from build123d import *

# Parameters (mm, degrees)
F1_DEPTH = 2.54
F2_DEPTH = 5.08
F3_DEPTH = 7.62


with BuildPart() as f1:
    # F0 (on Top) → F1 (new body)
    with BuildSketch(Plane.XY):
        Polygon((-24.428534, 7.051245), (-30.778534, -3.947278), (-28.57883, -5.217278), (-24.428534, 1.971245), (-20.278239, -5.217278), (-18.078534, -3.947278), align=None)
    extrude(amount=F1_DEPTH)

    # F0 (on Top) → F2 (join)
    with BuildSketch(Plane.XY):
        Polygon((-24.428534, -12.4058), (-24.428534, -14.9458), (-11.728534, -14.9458), (-18.078534, -3.947278), (-20.278239, -5.217278), (-16.127943, -12.4058), align=None)
    extrude(amount=F2_DEPTH)

    # F0 (on Top) → F3 (join)
    with BuildSketch(Plane.XY):
        Polygon((-30.778534, -3.947278), (-37.128534, -14.9458), (-24.428534, -14.9458), (-24.428534, -12.4058), (-32.729125, -12.4058), (-28.57883, -5.217278), align=None)
    extrude(amount=F3_DEPTH)


solid = f1.part
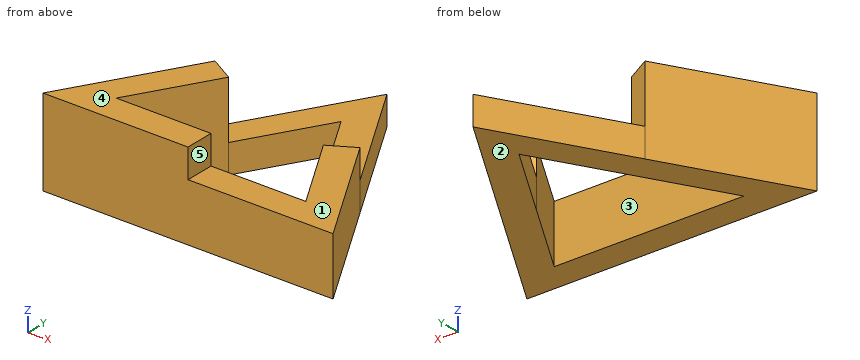
Model file for the job. Use its own axes, mm. Face numbers are marked on the shaded views. A direction names the side the tool comes from. Round coordinates to 2 decimals unless told otherwise and drop trailing zeros. Loops run counter-clockwise (first coordinate to the right, second up) from the corner with the lowest first, then second, coordinate; pieces in that order, holes last.
1. Band-saw the part on D-D, the plane z = 5.5. List the corners of the cut face in (x, y).
Check values:
outline: (-37.13, -14.95) - (-24.43, -14.95) - (-24.43, -12.41) - (-32.73, -12.41) - (-28.58, -5.22) - (-30.78, -3.95) - close
2. Tool access for the marked faces 1 and 2: list every direction of +Z, -Z, +X, -X, +Y, -Y with a clear straight run to the whole face (end or side of a thin tool).
Check values:
face 1: +Z, +X, +Y, -Y
face 2: -Z, +X, -X, +Y, -Y
3. Drop flat-ended pins along their axis: P1, Ø8, axis at x = -21, y = -7, coming from the +Z side; P2, Ø0.8, axis at y = -13.5, z = 6.5, coming from the +X side; P3, Ø4, axis at x = -26.5, z = 2.5, coming from the +Y side. Give the stop position or say it passes through.
Check values:
P1: stops at z = 5.08
P2: stops at x = -24.43
P3: stops at y = 6.93
4. Band-saw the part on C-C, the plane y = -2.5. List the corners of the cut face in (x, z), and give its area (3 significant figures).
Check values:
outline: (-29.94, 0) - (-27.01, 0) - (-27.01, 2.54) - (-29.94, 2.54) - close; (-21.85, 0) - (-18.91, 0) - (-18.91, 2.54) - (-21.85, 2.54) - close
area: 14.9 mm2
5. Wall check: probe 1 along Y at (x, z) = (-30, 1); probe 2 along Y at (x, z) = (-22, 3); probe 3 along Z at (x, y) = (-19.5, -2.75). Give the ranges that are in metal, low to high.
Check values:
probe 1: y = -14.95 to -12.41, -7.68 to -2.6
probe 2: y = -14.95 to -12.41
probe 3: z = 0 to 2.54
6. Band-saw the part on A-A, the plane x = -31.5. List the corners of the cut face in (y, z), and give its area (3 significant figures).
Check values:
outline: (-14.95, 0) - (-12.41, 0) - (-12.41, 7.62) - (-14.95, 7.62) - close; (-10.28, 0) - (-5.2, 0) - (-5.2, 7.62) - (-10.28, 7.62) - close
area: 58.1 mm2
7. Band-saw the part on B-B, the plane z = 2. List the corners of the cut face in (x, y), and give its area (3 significant figures).
Check values:
outline: (-37.13, -14.95) - (-11.73, -14.95) - (-24.43, 7.05) - close; hole (-32.73, -12.41) - (-16.13, -12.41) - (-20.28, -5.22) - (-24.43, 1.97) - close
area: 160 mm2
8. Mould opens along X. For the marked faces 3, 4 and 5 say: +X half, -X half, draft (parallel to the pull), parting line (faces both ways), or undercut.
Check values:
face 3: undercut
face 4: draft
face 5: +X half
